Could you check a few things on this model? Use its own coordinates, in mm. Face numbers are marked on the shaded views. A direction names the side the tool comes from. Give positions to 0.01 mm unless a question says otherwise; leave off trailing zeros. Order: outer loops, then holes, each group sorted by start corner. A loop starts at its lowest first (then second) coordinate and runs counter-clockwise, first axis right, second up. Notation, with made-up numbers: (-5, -15.75) -> (26, -15.75) arc R25 ccw to (26, 12.25) -> close; hole circle Ø2 at (16, 62). An arc over 180 degrees is marked (long way). One line per item, written item: value.
```python
from build123d import *

# Parameters (mm, degrees)
SKETCH2_R               = 6.35
BOSS_EXTRUDE1_DEPTH     = 6.35
SKETCH3_R               = 5.6388
BOSS_EXTRUDE2_DEPTH     = 15.113
SKETCH4_W               = 5.588
SKETCH4_H               = 1.17475
CUT_EXTRUDE1_DEPTH      = 6.35
F_1_4_28_TAPPED_HOLE1_D = 5.4102


with BuildPart() as part:
    # Sketch2 → Boss-Extrude1 (new body)
    with BuildSketch(Plane(origin=(0, 0, 0), x_dir=(0, 0, -1), z_dir=(1, 0, 0))):
        Circle(SKETCH2_R)
    extrude(amount=-BOSS_EXTRUDE1_DEPTH)

    # Sketch3 → Boss-Extrude2 (add)
    with BuildSketch(Plane(origin=(0, 0, 0), x_dir=(0, 0, -1), z_dir=(1, 0, 0))):
        Circle(SKETCH3_R)
    extrude(amount=BOSS_EXTRUDE2_DEPTH)

    # Sketch4 → Cut-Extrude1 (cut, symmetric)
    with BuildSketch(Plane(origin=(0, 0, 0), x_dir=(1, 0, 0), z_dir=(0, 1, 0))):
        with Locations((-3.556, 5.762625)):
            Rectangle(SKETCH4_W, SKETCH4_H)
        with Locations((-3.556, -5.762625)):
            Rectangle(SKETCH4_W, SKETCH4_H)
    extrude(amount=CUT_EXTRUDE1_DEPTH, both=True, mode=Mode.SUBTRACT)

    # 1/4-28 Tapped Hole1 (through all)
    with Locations(Plane(origin=(-6.35, 0, 0), x_dir=(0, 0, -1), z_dir=(-1, 0, 0))):
        with Locations((0, 0)):
            Hole(F_1_4_28_TAPPED_HOLE1_D / 2)


solid = part.part
```
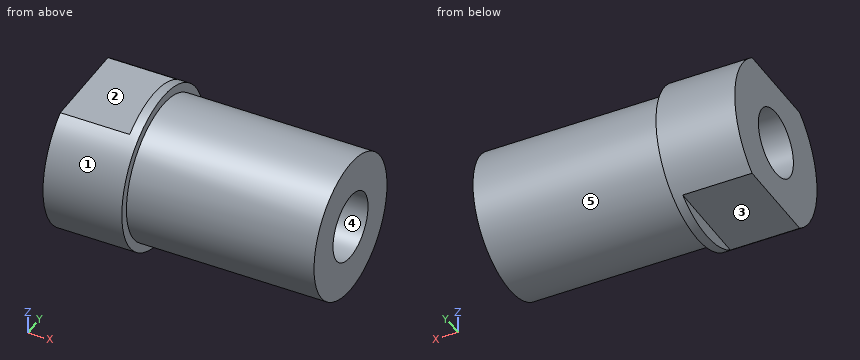
1) For the marked faces 1 and 2, which set-ups out of +Z, -Z, +X, -X, +Y, -Y let a thin tool reach every point of the face, with its end or its side?
Answer below:
face 1: +X, -X
face 2: +Z, -X, +Y, -Y
2) Suppose I cut it at A-A, the plane z = 0. Write out the boundary of the cut face in (x, y).
Answer below:
outline: (-6.35, -6.35) -> (0, -6.35) -> (0, -5.64) -> (15.11, -5.64) -> (15.11, -2.71) -> (-6.35, -2.71) -> close; (-6.35, 2.71) -> (15.11, 2.71) -> (15.11, 5.64) -> (0, 5.64) -> (0, 6.35) -> (-6.35, 6.35) -> close
3) Suppose I cut it at C-C, the plane x = 2.5. Write out the boundary of the cut face in (y, z), then the cut area to 3 significant figures.
Answer below:
outline: circle Ø11.28 at (0, 0); hole circle Ø5.41 at (0, 0)
area: 76.9 mm2
4) For P1, Ø6, axis at x = 11.5, y = -2.5, coming from the +Z side; P2, Ø1.7, axis at x = -4.5, y = -1.5, coming from the -Z side; P3, Ø6, axis at x = -5, y = 1.5, coming from the +Z side, each with a flat end and sliding along its axis, tell me the tip position at first contact or that it passes through.
Answer below:
P1: stops at z = 5.64
P2: stops at z = -5.18
P3: stops at z = 5.18
5) We'd pull the mould along Y, two halves only. Please class the marked faces 3, 4 and 5: +Y half, -Y half, draft (parallel to the pull), parting line (faces both ways), or undercut.
Answer below:
face 3: draft
face 4: undercut
face 5: parting line
6) Suppose I cut it at D-D, the plane y = 3. Write out the boundary of the cut face in (x, z), then the cut area to 3 significant figures.
Answer below:
outline: (-6.35, -5.18) -> (-0.76, -5.18) -> (-0.76, -5.6) -> (0, -5.6) -> (0, -4.77) -> (15.11, -4.77) -> (15.11, 4.77) -> (0, 4.77) -> (0, 5.6) -> (-0.76, 5.6) -> (-0.76, 5.18) -> (-6.35, 5.18) -> close
area: 211 mm2
7) If I drill on line 1 along Y through (x, z) = (8.25, 0); line 2 along X through (y, z) = (3.5, 5.25); line 3 along Z through (x, y) = (4.5, 2.25), over which ranges is the centre line in solid material (lowest first)?
Answer below:
line 1: y = -5.64 to -2.71, 2.71 to 5.64
line 2: x = -0.76 to 0
line 3: z = -5.17 to -1.5, 1.5 to 5.17
8) Suppose I cut it at B-B, the plane y = 0. Write out the boundary of the cut face in (x, z).
Answer below:
outline: (-6.35, -5.18) -> (-0.76, -5.18) -> (-0.76, -6.35) -> (0, -6.35) -> (0, -5.64) -> (15.11, -5.64) -> (15.11, -2.71) -> (-6.35, -2.71) -> close; (-6.35, 2.71) -> (15.11, 2.71) -> (15.11, 5.64) -> (0, 5.64) -> (0, 6.35) -> (-0.76, 6.35) -> (-0.76, 5.18) -> (-6.35, 5.18) -> close
